Input: dimensioned drawing with shaded views. Units: mm. Origin: part minimum x, y, z. Coordinates: 2 decimals unless noted, no trailing zeros. Loops run counter-clockwise (first coordinate to the right, second up) from the corner with the lowest first, then second, coordinate; pieces in that order, holes last.
Item 1: Section C-C on z = 3.9. Return loops of the section in (x, y), and give its area (3 significant figures).
Item 2: Contact query for flat-ended pins moving along their axis: P1, Ø1.5, axis at x = 1.5, z = 1, coming from the -Y side; P2, Ø3.5, axis at x = 3.9, z = 3.9, coming from the +Y side. Output: stop coordinate, or through.
Item 3: Section A-A on x = 3.9. Return loops of the section in (y, z).
Item 4: Section D-D on y = 1. Return loops of the section in (x, z), and give its area (3 significant figures).
Item 5: Section B-B on y = 0.5. Return loops of the section in (x, z).
Item 6: Pull-direction query (X, two-part tool) for the marked faces 1 and 2; classes: released by +X, released by -X, zero draft, split by the parting line, or undercut.
Item 7: Ray query, line 1 along X through (y, z) = (0.35, 3.9); line 2 along Z through (x, y) = (4.75, 0.5); line 3 along X through (y, z) = (0.4, 2.25). Return the intervals inside material, ascending.
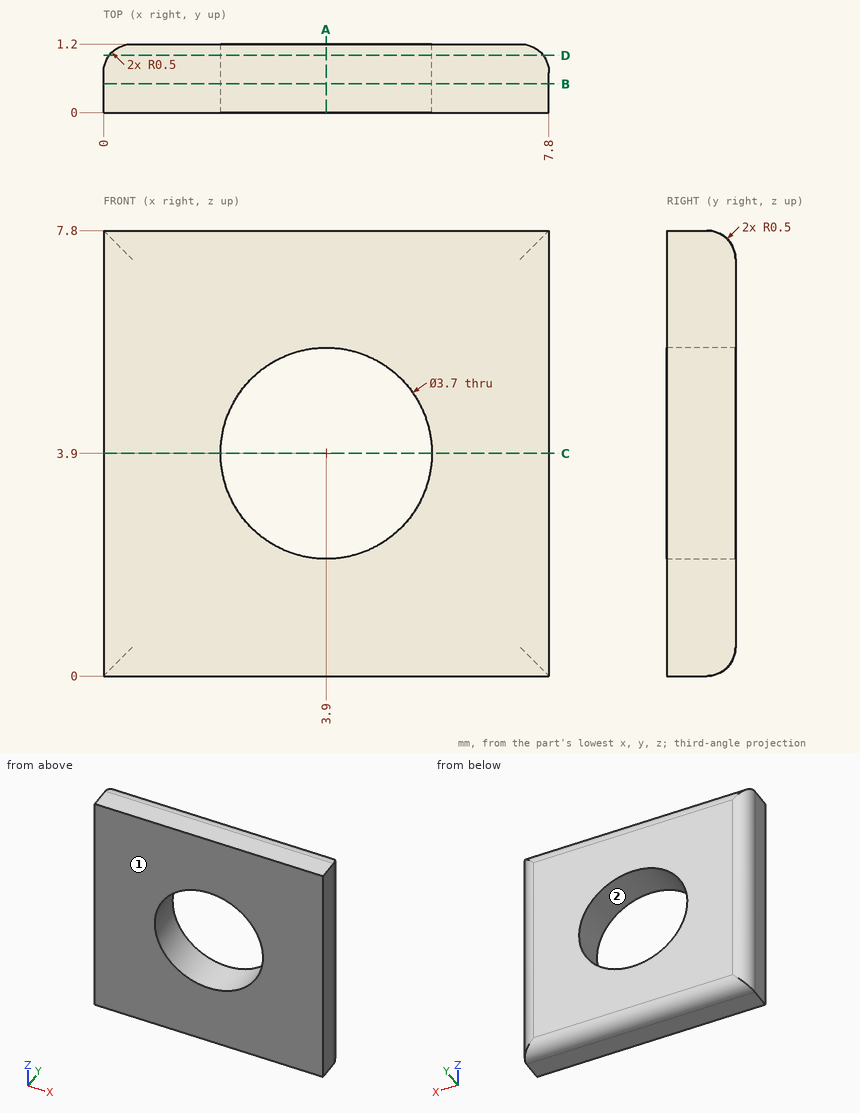
Results found:
1. outline: (0, 0) - (2.05, 0) - (2.05, 1.2) - (0.5, 1.2) arc R0.5 ccw to (0, 0.7) - close; (5.75, 0) - (7.8, 0) - (7.8, 0.7) arc R0.5 ccw to (7.3, 1.2) - (5.75, 1.2) - close
1. area: 4.81 mm2
2. P1: stops at y = 0
2. P2: passes through
3. outline: (0, 0) - (0.7, 0) arc R0.5 ccw to (1.2, 0.5) - (1.2, 2.05) - (0, 2.05) - close; (0, 5.75) - (1.2, 5.75) - (1.2, 7.3) arc R0.5 ccw to (0.7, 7.8) - (0, 7.8) - close
4. outline: (0.1, 0.1) - (7.7, 0.1) - (7.7, 7.7) - (0.1, 7.7) - close; hole circle Ø3.7 at (3.9, 3.9)
4. area: 47.0 mm2
5. outline: (0, 0) - (7.8, 0) - (7.8, 7.8) - (0, 7.8) - close; hole circle Ø3.7 at (3.9, 3.9)
6. face 1: zero draft
6. face 2: undercut
7. line 1: x = 0 to 2.05, 5.75 to 7.8
7. line 2: z = 0 to 2.26, 5.54 to 7.8
7. line 3: x = 0 to 3.06, 4.74 to 7.8
